from build123d import *

# Parameters (mm, degrees)
SKETCH_1_W                  = 70
SKETCH_1_H                  = 100
EXTRUDE_1_DEPTH             = 4
SKETCH_2_R                  = 5
EXTRUDE_2_DEPTH             = 3
SKETCH_3_R                  = 1.9
CUT_EXTRUDE_1_DEPTH         = 4
SKETCH_6_R                  = 2.1
CUT_EXTRUDE_4_DEPTH         = 5
PATTERN_LINEAR_1_COUNT      = 3
PATTERN_LINEAR_1_PITCH      = 20
PATTERN_LINEAR_1_COUNT_DIR2 = 4
PATTERN_LINEAR_1_PITCH_DIR2 = 20
CUT_EXTRUDE_START           = -5
CUT_EXTRUDE_5_DEPTH         = 9
CHAMFER_1_SIZE              = 5
FILLET_1_R                  = 10


with BuildPart() as part:
    # 草圖1 → 填料-伸長1 (new body)
    with BuildSketch(Plane(origin=(0, 0, 0), x_dir=(1, 0, 0), z_dir=(0, 1, 0))):
        Rectangle(SKETCH_1_W, SKETCH_1_H)
    extrude(amount=EXTRUDE_1_DEPTH)

    # 草圖2 → 填料-伸長2 (add)
    with BuildSketch(Plane(origin=(0, 4, 0), x_dir=(1, 0, 0), z_dir=(0, 1, 0))):
        with Locations((-22.1, 40)):
            Circle(SKETCH_2_R)
        with Locations((22.1, 40)):
            Circle(SKETCH_2_R)
        with Locations((0, -40)):
            Circle(SKETCH_2_R)
    extrude(amount=EXTRUDE_2_DEPTH)

    # 草圖3 → 除料-伸長1 (cut)
    with BuildSketch(Plane(origin=(0, 7, 0), x_dir=(1, 0, 0), z_dir=(0, 1, 0))):
        with Locations((-22.1, 40)):
            Circle(SKETCH_3_R)
        with Locations((22.1, 40)):
            Circle(SKETCH_3_R)
        with Locations((0, -40)):
            Circle(SKETCH_3_R)
    extrude(amount=-CUT_EXTRUDE_1_DEPTH, mode=Mode.SUBTRACT)

    # 草圖6 → 除料-伸長4 (cut, through all)
    with BuildSketch(Plane(origin=(0, 4, 0), x_dir=(1, 0, 0), z_dir=(0, 1, 0))):
        with Locations((-20, 30)):
            Circle(SKETCH_6_R)
    cut_extrude_4 = extrude(amount=-CUT_EXTRUDE_4_DEPTH, mode=Mode.SUBTRACT)

    # 直線複製排列1: Cut-Extrude 4 3 × 4, 6 skipped
    with Locations(*[(i * PATTERN_LINEAR_1_PITCH, 0, j * PATTERN_LINEAR_1_PITCH_DIR2) for i in range(PATTERN_LINEAR_1_COUNT) for j in range(PATTERN_LINEAR_1_COUNT_DIR2) if (i, j) not in ((0, 0), (0, 1), (0, 2), (1, 1), (1, 2), (2, 1), (2, 2))]):
        add(cut_extrude_4, mode=Mode.SUBTRACT)

    # 草圖7 → 除料-伸長5 (cut)
    with BuildSketch(Plane(origin=(0, 4, 0), x_dir=(1, 0, 0), z_dir=(0, 1, 0)).offset(CUT_EXTRUDE_START)):
        Polygon((-35, 30), (-15, 20), (-15, -20), (-35, -30), align=None)
    cut_extrude_5 = extrude(amount=CUT_EXTRUDE_5_DEPTH, mode=Mode.SUBTRACT)

    # 鏡射1: 除料-伸長5 across plane
    add(cut_extrude_5.mirror(Plane(origin=(0, 0, 0), x_dir=(0, 0, 1), z_dir=(1, 0, 0))), mode=Mode.SUBTRACT)

    # 導角1
    chamfer_1_edges = [part.edges().sort_by_distance(p)[0] for p in [
        (35, 2, 50),
        (-35, 2, 50),
        (-35, 2, -50),
        (35, 2, -50),
    ]]
    chamfer(chamfer_1_edges, length=CHAMFER_1_SIZE)

    # 圓角1
    fillet_1_edges = [part.edges().sort_by_distance(p)[0] for p in [
        (-15, 2, -20),
        (-15, 2, 20),
        (15, 2, 20),
        (15, 2, -20),
    ]]
    fillet(fillet_1_edges, radius=FILLET_1_R)


solid = part.part
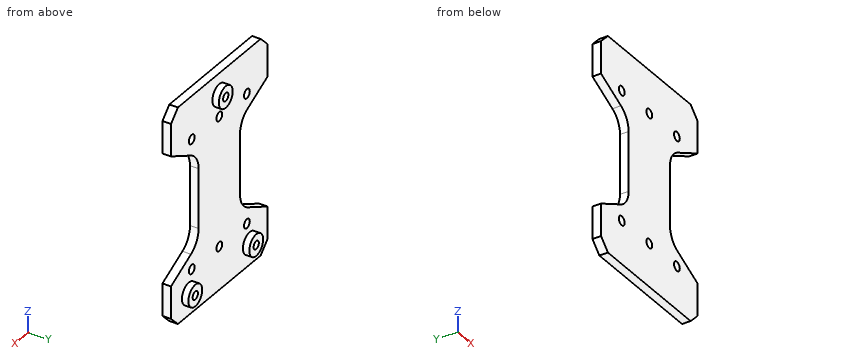
Work out the finished part from the listing and answer in its coordinate system (mm). Give positions to 0.01 mm unless a question says otherwise; leave off trailing zeros. Loops run counter-clockwise (first coordinate to the right, second up) from the corner with the lowest first, then second, coordinate; pieces in that order, holes last. Notation, with made-up numbers: (40.5, 69.25) -> (85.5, 69.25) arc R24 ccw to (85.5, 103.25) -> close; hole circle Ø6 at (-24, 12.5). An arc over 180 degrees is marked (long way). Use a Markdown table: item, result. Add a question column.
1) Consider line 1 along Z through (x, y) = (0, 1.6); line 2 along X through (y, z) = (5.95, -40); line 3 along X through (y, z) = (0.5, 30). Determine where each line is inside the solid, lowest interval first.
2) The part is cut by section B-B, the plane x = 0. Determine the outline of the cut face in (y, z).
3) The part is cut by section D-D, the plane z = 40. Determine the outline of the cut face in (x, y), plus the area to 3 significant figures.
4) Each of these flat-tipped pins is pushed along its axis until it touches: P1, Ø3, axis at x = 22.1, z = -40, coming from the +Y side; P2, Ø1.9, axis at x = -21, z = -40.5, coming from the +Y side; P3, Ø5, axis at x = 0, z = 30, coming from the +Y side; P4, Ø2, axis at x = -20.5, y = 5.5, coming from the -Z side. Where does it stop, or does it pass through?
5) The part is cut by section A-A, the plane y = 5. Determine the outline of the cut face in (x, z).
6) The part is cut by section C-C, the plane z = -44. Determine the outline of the cut face in (x, y).
Reported:
| question | item | result |
|---|---|---|
| 1 | line 1 | z = -50 to -32.1, -27.9 to 27.9, 32.1 to 50 |
| 1 | line 2 | x = -27.1 to -24, -20.2 to -17.1, 17.1 to 20.2, 24 to 27.1 |
| 1 | line 3 | x = -35 to -22.1, -17.9 to -2.1, 2.1 to 17.9, 22.1 to 35 |
| 2 | outline | (0, -50) -> (4, -50) -> (4, -32.1) -> (0, -32.1) -> close; (0, -27.9) -> (4, -27.9) -> (4, 27.9) -> (0, 27.9) -> close; (0, 32.1) -> (4, 32.1) -> (4, 35) -> (7, 35) -> (7, 38.1) -> (3, 38.1) -> (3, 41.9) -> (7, 41.9) -> (7, 45) -> (4, 45) -> (4, 50) -> (0, 50) -> close |
| 3 | outline | (-35, 0) -> (35, 0) -> (35, 4) -> (5, 4) -> (5, 7) -> (1.9, 7) -> (1.9, 3) -> (-1.9, 3) -> (-1.9, 7) -> (-5, 7) -> (-5, 4) -> (-35, 4) -> close |
| 3 | area | 295 mm^2 |
| 4 | P1 | stops at y = 3 |
| 4 | P2 | stops at y = 7 |
| 4 | P3 | stops at y = 4 |
| 4 | P4 | stops at z = -44.96 |
| 5 | outline | circle Ø10 at (-22.1, -40); circle Ø10 at (0, 40); circle Ø10 at (22.1, -40); hole circle Ø3.8 at (-22.1, -40); hole circle Ø3.8 at (0, 40); hole circle Ø3.8 at (22.1, -40) |
| 6 | outline | (-35, 0) -> (35, 0) -> (35, 4) -> (25.1, 4) -> (25.1, 7) -> (19.1, 7) -> (19.1, 4) -> (-19.1, 4) -> (-19.1, 7) -> (-25.1, 7) -> (-25.1, 4) -> (-35, 4) -> close |
